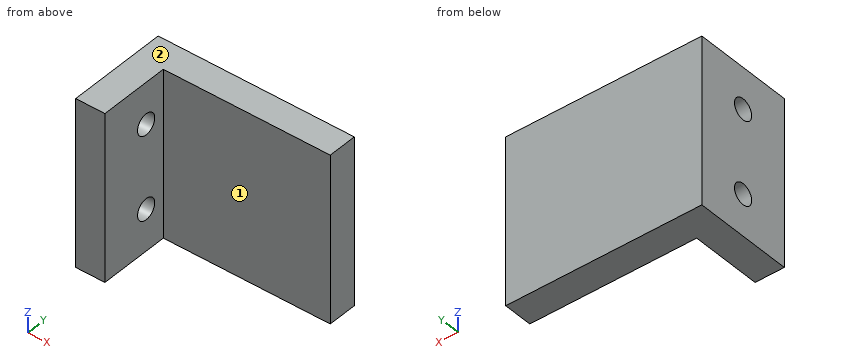
```python
from build123d import *

# Parameters (mm, degrees)
SKETCH1_W           = 40
SKETCH1_H           = 24
BOSS_EXTRUDE1_DEPTH = 7
SKETCH2_W           = 40
SKETCH2_H           = 7
BOSS_EXTRUDE2_DEPTH = 40
SKETCH3_R           = 2.5
CUT_EXTRUDE1_DEPTH  = 14


with BuildPart() as part:
    # Sketch1 → Boss-Extrude1 (new body)
    with BuildSketch(Plane(origin=(0, 0, 0), x_dir=(0, 0, -1), z_dir=(1, 0, 0))):
        Rectangle(SKETCH1_W, SKETCH1_H)
    extrude(amount=BOSS_EXTRUDE1_DEPTH)

    # Sketch2 → Boss-Extrude2 (add)
    with BuildSketch(Plane(origin=(7, 0, 0), x_dir=(0, 0, -1), z_dir=(1, 0, 0))):
        with Locations((0, 8.5)):
            Rectangle(SKETCH2_W, SKETCH2_H)
    extrude(amount=BOSS_EXTRUDE2_DEPTH)

    # Sketch3 → Cut-Extrude1 (cut)
    with BuildSketch(Plane.ZY):
        with Locations((-10.048887394, 0)):
            Circle(SKETCH3_R)
        with Locations((10.048887394, 0)):
            Circle(SKETCH3_R)
    extrude(amount=-CUT_EXTRUDE1_DEPTH, mode=Mode.SUBTRACT)


solid = part.part
```
Check sheet for the modelled part. Datum: model origin and axes. Units: mm. Face numbers are marked on the shaded views. A direction names the side the tool comes from. Give positions to 0.01 mm unless a question says otherwise; leave off trailing zeros. Write each loop counter-clockwise with the first axis right and the second up, starting at its lowest first coordinate (ties: lowest second). Pieces come first, ordered by that corner, then holes. Notation, with made-up numbers: (8, 9) - (58, 9) arc R21 cw to (58, 45) - close; hole circle Ø9 at (76.25, 44). An arc over 180 degrees is marked (long way). Answer as a JSON object with one key per item and string values. Group by question number.
1) Sectioned sample at D-D (z = 1). Record the cut outline in (x, y).
2) Depth check by flat-ended pin: P1, Ø1, axis at x = 13.5, z = 12.5, coming from the -Y side; P2, Ø6, axis at y = 0, z = -10.05, coming from the +X side; P3, Ø1.5, axis at y = 0.5, z = 1.5, coming from the -X side. Enter the tip coordinate at first touch or a pass-through.
3) Thickness scan on probe 1 along Y at (x, z) = (10.5, 2); probe 2 along X at (y, z) = (-5.5, -13). Record the ranges inside material, lowest first. Write a range as from..to.
4) Sectioned sample at B-B (z = 12). Record the cut outline in (x, y), then the cut area to 3 significant figures.
5) Access from +Z, -Z, +X, -X, +Y, -Y to the whole of each face (thin tool, end or side, straight path). Record for the marked faces 1 and 2.
6) Sectioned sample at A-A (y = 0). Record the cut outline in (x, z), then the cut area to 3 significant figures.
7) Sectioned sample at C-C (x = 39). Record the cut outline in (y, z), then the cut area to 3 significant figures.
Geometry results:
{
 "1": {"outline": "(0, -12) - (7, -12) - (7, 5) - (47, 5) - (47, 12) - (0, 12) - close"},
 "2": {"P1": "stops at y = 5", "P2": "stops at x = 7", "P3": "stops at x = 0"},
 "3": {"probe 1": "y = 5..12", "probe 2": "x = 0..7"},
 "4": {"outline": "(0, -12) - (7, -12) - (7, -1.56) - (0, -1.56) - close; (0, 1.56) - (7, 1.56) - (7, 5) - (47, 5) - (47, 12) - (0, 12) - close", "area": "426 mm^2"},
 "5": {"face 1": "+Z, -Z, +X, -Y", "face 2": "+Z, +X, -X, +Y, -Y"},
 "6": {"outline": "(0, -20) - (7, -20) - (7, -12.55) - (0, -12.55) - close; (0, -7.55) - (7, -7.55) - (7, 7.55) - (0, 7.55) - close; (0, 12.55) - (7, 12.55) - (7, 20) - (0, 20) - close", "area": "210 mm^2"},
 "7": {"outline": "(5, -20) - (12, -20) - (12, 20) - (5, 20) - close", "area": "280 mm^2"}
}
